```python
from build123d import *

# Parameters (mm, degrees)
F0_W      = 31.75
F0_H      = 29.21
F0_R      = 14.2875
F0_R_2    = 13.335
F0_R_3    = 7.9375
F0_R_4    = 1.6383
F1_DEPTH  = 25.4
F2_R      = 6.1214
F2_R_2    = 1.6383
F3_DEPTH  = 9.525
F4_R      = 3.175
F4_R_2    = 1.6383
F5_DEPTH  = 1.27
F7_DEPTH  = 21.59
F8_SIZE   = 0.635
F9_R      = 7.9375
F10_DEPTH = 12.7
F11_R     = 1.1938
F12_DEPTH = 6.35
F13_R     = 1.190625
F14_DEPTH = 31.751
F17_R     = 7.9375
F18_DEPTH = 12.7
F19_R     = 9.7155
F20_DEPTH = 0.762


# Not quite as in the source:
# - a feature names something its author has since deleted; it is built from what else it names


with BuildPart() as f1:
    # F0 (on Top) → F1 (new body)
    with BuildSketch(Plane.XY):
        Rectangle(F0_W, F0_H)
        Circle(F0_R, mode=Mode.SUBTRACT)
        Circle(F0_R)
        Circle(F0_R_2, mode=Mode.SUBTRACT)
        Circle(F0_R_2)
        Circle(F0_R_3, mode=Mode.SUBTRACT)
        Circle(F0_R_3)
        Circle(F0_R_4, mode=Mode.SUBTRACT)
    extrude(amount=F1_DEPTH)

    # F2 (on face) → F3 (join)
    with BuildSketch(Plane.XY.offset(25.4)):
        Circle(F2_R)
        Circle(F2_R_2, mode=Mode.SUBTRACT)
    extrude(amount=F3_DEPTH)

    # F4 (on face) → F5 (cut)
    with BuildSketch(Plane.XY.offset(34.925)):
        Circle(F4_R)
        Circle(F4_R_2, mode=Mode.SUBTRACT)
    extrude(amount=-F5_DEPTH, mode=Mode.SUBTRACT)

    # F0 (on Top) → F7 (cut)
    with BuildSketch(Plane.XY):
        Circle(F0_R_3)
        Circle(F0_R_4, mode=Mode.SUBTRACT)
    extrude(amount=F7_DEPTH, mode=Mode.SUBTRACT)

    # F8
    f8_edges = [f1.edges().sort_by_distance(p)[0] for p in [
        (-6.1214, 0, 34.925),
    ]]
    chamfer(f8_edges, length=F8_SIZE)

    # F9 (on face) → F10 (cut)
    with BuildSketch(Plane.XZ.offset(14.605)):
        with Locations((0, 12.7)):
            Circle(F9_R)
    extrude(amount=-F10_DEPTH, mode=Mode.SUBTRACT)

    # F11 (on face) → F12 (cut)
    with BuildSketch(Plane(origin=(0, 14.605, 0), x_dir=(-1, 0, 0), z_dir=(0, 1, 0))):
        with Locations((0, 12.7)):
            Circle(F11_R)
    extrude(amount=-F12_DEPTH, mode=Mode.SUBTRACT)

    # F13 (on face) → F14 (cut, through all)
    with BuildSketch(Plane.YZ.offset(15.875)):
        with Locations((-5.08, 12.7)):
            Circle(F13_R)
    extrude(amount=-F14_DEPTH, mode=Mode.SUBTRACT)

    # F15 (on Front) → F16 (revolve)
    with BuildSketch(Plane.XZ):
        Polygon((0, 0), (0, -12.7), (13.335, -12.7), (13.335, -11.1125), (12.065, -11.1125), (12.065, -8.6995), (13.335, -8.6995), (13.335, -0.508), (14.2875, -0.508), (14.2875, 0), align=None)
    revolve(axis=Axis((0, 0, -6.35), (0, 0, -1)))

    # F17 (on face) → F18 (cut)
    with BuildSketch(Plane(origin=(0, 0, -12.7), x_dir=(1, 0, 0), z_dir=(0, 0, -1))):
        Circle(F17_R)
    extrude(amount=-F18_DEPTH, mode=Mode.SUBTRACT)

    # F19 (on face) → F20 (cut)
    with BuildSketch(Plane(origin=(0, 0, -12.7), x_dir=(1, 0, 0), z_dir=(0, 0, -1))):
        Circle(F19_R)
    extrude(amount=-F20_DEPTH, mode=Mode.SUBTRACT)


solid = f1.part
```
The listing builds one solid part. Answer for the finished solid, in the listing's coordinates (mm). A direction names the side the tool comes from. Give positions to 0.01 mm unless a question says otherwise; leave off trailing zeros. Order: outer loops, then holes, each group sorted by start corner. A loop starts at its lowest first (then second) coordinate and runs counter-clockwise, first axis right, second up. Notation, with made-up numbers: (86, 39.5) - (108, 39.5) arc R23 ccw to (108, 76.5) - close; hole circle Ø1 at (65, 37.5). An arc over 180 degrees is marked (long way). Use one line per item in the form item = value. Start each with the question number.
(1) A cutting plane is placed at D-D, the plane z = 6. Write down the section's boundary in (x, y) (1 decimal).
(2) A cutting plane is placed at B-B, the plane z = -7. Write down the section's boundary in (x, y) (1 decimal), then the cut area to 3 significant figures.
(3) The mould has two halves that part along Z. Classify faces 6 (the flat face through (2.4, -2.4, 34.925)), 7 (the cylindrical face through (11.918, -3.944, 13.058)), 8 (the flat face through (15.875, 0, 13)): released by +Z, released by -Z, zero draft, split by the parting line, or undercut.
(4) Flat-ended cylindrical pins translate along their axes: pin 1 Ø14.5 at (x, y) = (3, 4.5) entering from -Z; pin 2 Ø3 at (y, z) = (5, 27) entering from +X; pin 3 Ø8 at (x, y) = (0.5, 5) entering from -Z; pin 4 Ø3 at (x, z) = (0, 12.7) entering from -Y. Find the tip coordinate at first contact, or state that the pin passes through.
(5) A cutting plane is placed at A-A, the plane z = 12.7. State how many separate pieces and enclosed holes the cut face has, then the cut area to 3 significant figures.
(6) Consider line 1 (Y direction, x = 0, z = -12.3) (1 decimal); line 2 (Z direction, x = -0.5, y = 12.25); line 3 (X direction, y = -8, z = 12.7) (1 decimal). Determine where each line is inside the solid, lowest interval first. Write a range as from..to.
(7) For faces 1 (the cylindrical face through (-14.274, -0.628, -0.25)), 2 (the flat face through (0, 8.255, 13)), 3 (the cylindrical face through (-0.69, -3.1, 34.3)), 4 (the cylindrical face through (7.571, -9.755, 15.084)), 5 (the flat face through (3, 12, -8.7)), determine the directions among +Z, -Z, +X, -X, +Y, -Y from which every point of the face is accessible in a straight line to the end or side of a thin tool.
Ans:
q1.outline = (-15.9, -14.6) - (-4.3, -14.6) - (-4.3, -6.7) arc R7.9 cw (long way) to (4.3, -6.7) - (4.3, -14.6) - (15.9, -14.6) - (15.9, 14.6) - (-15.9, 14.6) - close
q2.outline = circle Ø26.7 at (0, 0); hole circle Ø15.9 at (0, 0)
q2.area = 361 mm^2
q3.face_6 = released by +Z
q3.face_7 = undercut
q3.face_8 = zero draft
q4.pin_1 = -12.7
q4.pin_2 = 5.02
q4.pin_3 = -11.94
q4.pin_4 = 7.79
q5.separate_pieces = 3
q5.enclosed_holes = 0
q5.area = 544 mm^2
q6.line_1 = -13.3..-9.7, 9.7..13.3
q6.line_2 = -12.7..-11.11, -8.7..11.62, 13.78..25.4
q6.line_3 = -15.9..-7.9, 7.9..15.9
q7.face_1 = -Z
q7.face_2 = +Y
q7.face_3 = +Z
q7.face_4 = -Y
q7.face_5 = none
